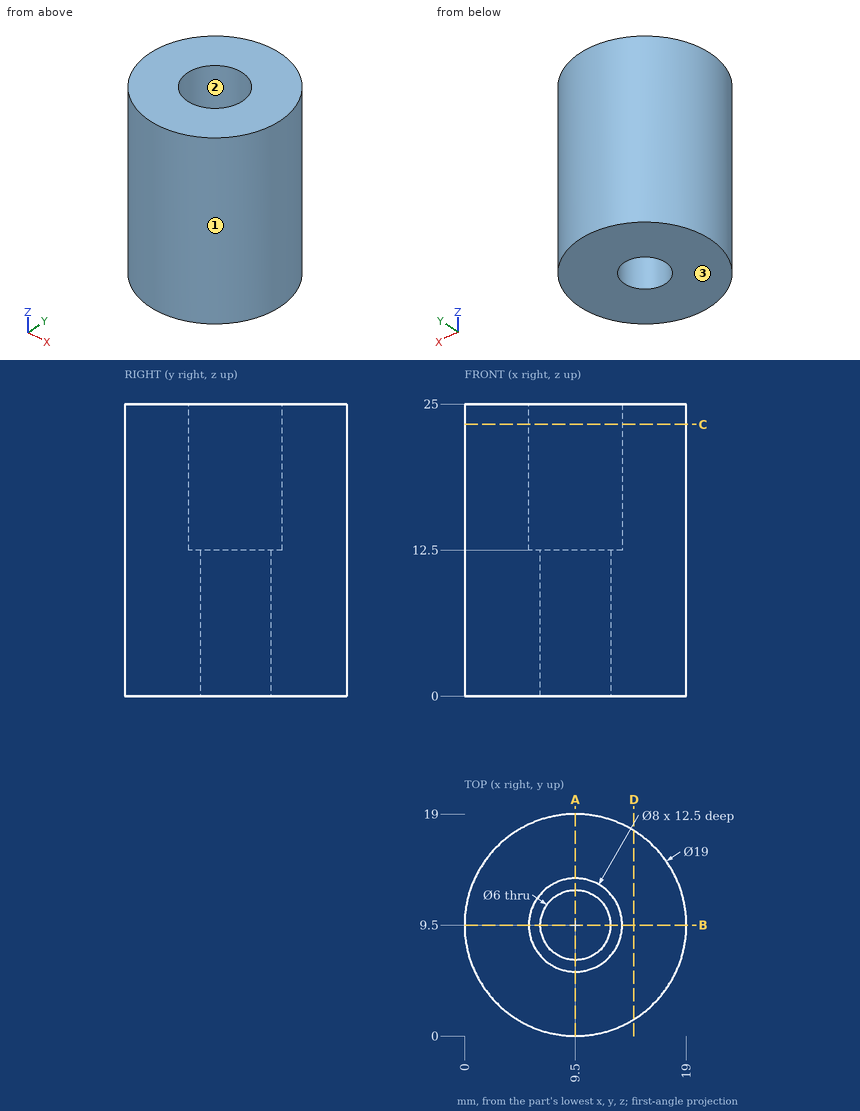
Here's the drawing with two shaded views (mm, measured from the low corner). I have some questions. Round coordinates to 2 decimals unless told otherwise and drop trailing zeros. Loops run counter-clockwise (first coordinate to the right, second up) from the corner with the lowest first, then second, coordinate; pieces in that order, holes last. Notation, with made-up numbers: M 62.5,-8.75 L 77.5,-8.75 A28 cw 77.5,23.25 Z; hole C 33.5,68 d3. An arc over 180 degrees is marked long. Put each result on its own line as item: value.
Q1. Thinking about a two-plate mould opening in Y: for the marked faces 1, 2 and 3, which applies, released by +Y, released by -Y, zero draft, split by the parting line, or undercut?
Check result:
face 1: split by the parting line
face 2: undercut
face 3: zero draft
Q2. Imagine slicing it at D-D (x = 14.5). Write out the boundary of the cut face in (y, z).
Check result:
outline: M 1.42,0 L 17.58,0 L 17.58,25 L 1.42,25 Z
Q3. Imagine slicing it at A-A (x = 9.5). Write out the boundary of the cut face in (y, z).
Check result:
outline: M 0,0 L 6.5,0 L 6.5,12.5 L 5.5,12.5 L 5.5,25 L 0,25 Z; M 12.5,0 L 19,0 L 19,25 L 13.5,25 L 13.5,12.5 L 12.5,12.5 Z
Q4. I need wall thicknesses on probe 1 along Y at (x, z) = (9.5, 18); probe 2 along Y at (x, z) = (9.5, 5); probe 3 along X at (y, z) = (8.25, 6). Which ranges of each line are inside material? Lowest first, please.
Check result:
probe 1: 0 to 5.5, 13.5 to 19
probe 2: 0 to 6.5, 12.5 to 19
probe 3: 0.08 to 6.77, 12.23 to 18.92
Q5. For pin 1 (6 mm diameter, centred on y = 14.5, z = 6.5, fed in from -X); pin 2 (1.5 mm diameter, centred on x = 3.5, z = 16.5, fed in from -Y); pin 3 (3.5 mm diameter, centred on x = 9.5, y = 9.5, fed in from +Z); pin 4 (4 mm diameter, centred on y = 14, z = 10.5, fed in from +X), each with a flat end and sliding along its axis, tell me the tip position at first contact or that it passes through.
Check result:
pin 1: x = 0.21
pin 2: y = 1.58
pin 3: through
pin 4: x = 18.67
Q6. Imagine slicing it at C-C (z = 23.25). Write out the boundary of the cut face in (x, y).
Check result:
outline: C 9.5,9.5 d19; hole C 9.5,9.5 d8
